from build123d import *

# Parameters (mm, degrees)
SKETCH1_R = 1.27


with BuildPart() as part:
    # Sweep1: sweep along a curve in space
    with BuildLine() as sweep1_path:
        Line((-68.642810089, 4.223652332, 31.692711576), (-15.557895559, 0.136909795, 1.027320033))
        ThreePointArc((-15.557895559, 0.136909795, 1.027320033), (-13.708278185, 0.034830032, 0.261351566), (-11.721145923, 0, 0))
        Line((-11.721145923, 0, 0), (0, 0, 0))
    # Sketch1 → Sweep1 (sweep)
    with BuildSketch(Plane(origin=(-68.642810089, 4.223652332, 31.692711576), x_dir=(-0.4976253626044802, 0.038309692214518805, -0.8665456514086194), z_dir=(0.8639891352609107, -0.06651420995766534, -0.4990978200962329))):
        Circle(SKETCH1_R)
    sweep(path=sweep1_path.line)

    # Sketch2 → Revolve1 (revolve)
    with BuildSketch(Plane(origin=(-60.961946677, 3.632341006, 27.255731955), x_dir=(-0.4976253626044802, 0.038309692214518805, -0.8665456514086194), z_dir=(0.8639891352609107, -0.06651420995766534, -0.4990978200962329))):
        with BuildLine():
            Line((0, 2.54), (0, -2.54))
            ThreePointArc((0, -2.54), (2.54, 0), (0, 2.54))
        make_face()
    revolve(axis=Axis((-60.766981653, 6.164847401, 27.255731955), (-0.07675788326851926, -0.997049761725129, 0)))


solid = part.part
Build history of the part. All positions in model axes, mm. A direction names the side the tool comes from. Round coordinates to 2 decimals unless told otherwise and drop trailing zeros. Write item = value, one per line.
(1) Tool access for faces 1 (the face through (-65.08, 4.01, 31.1)), 2 (the face through (-5.779, -1.114, -0.609)): list every direction of +Z, -Z, +X, -X, +Y, -Y with a clear straight run to the whole face (end or side of a thin tool).
Answer:
face_1 = none
face_2 = +X
(2) Flat gauge pins, fed straight in: pin 1 (12 mm diameter, centred on x = -57.5, z = 25, fed in from +Y); pin 2 (3 mm diameter, centred on x = -10.5, y = 2.5, fed in from -Z); pin 3 (4 mm diameter, centred on y = 3.5, z = 23, fed in from -X); pin 4 (4 mm diameter, centred on y = 3, z = 22.5, fed in from +X). Where does each tip first touch, or does it go through?
Answer:
pin_1 = 6.17
pin_2 = -0.78
pin_3 = -62.13
pin_4 = -46.78
(3) Probe L1, parallel to Z at x = -56, y = 2.75; L2, parallel to Z at x = -28, y = 0.25. List the from-to ranges inside material, lowest first.
Answer:
L1 = 23.02 to 25.72
L2 = 7.08 to 9.27
